Solid Edge part; units mm, degrees
sketch "Sketch1" plane through (0, 0, 0) normal (0, 0, 1) x (1, 0, 0)
  circle A0 centre (0, 0) radius 4.25
extrude "Protrusion1" add sketch "Sketch1" along normal blind 5
sketch "Sketch2" plane through (0, 0, 0) normal (0, 0, -1) x (1, 0, 0)
  circle A0 centre (0, 0) radius 2.5
extrude "Protrusion2" add sketch "Sketch2" along normal blind 20
sketch "Sketch3" plane through (0, 0, -20) normal (0, 0, -1) x (1, 0, 0)
  circle A0 centre (0, 0) radius 2.4997
extrude "Cutout1" cut sketch "Sketch3" against normal blind 19.98 flip side to cut
chamfer "Chamfer_1" distance 0.375 angle 45 1 edges at (-2.4997, 0, -20)
sketch "Sketch4" plane through (0, 0, 5) normal (0, 0, 1) x (1, 0, 0)
  line L0 (-1.1547, 2) -> (1.1547, 2)
  line L1 (2.3094, 0) -> (1.1547, 2)
  line L2 (1.1547, -2) -> (2.3094, 0)
  line L3 (-1.1547, -2) -> (1.1547, -2)
  line L4 (-2.3094, 0) -> (-1.1547, -2)
  line L5 (-1.1547, 2) -> (-2.3094, 0)
extrude "Cutout2" cut sketch "Sketch4" against normal blind 2.5
properties part number "24104804"
Can you work these out from the model? Positions are in its coordinate system, mm. A direction names the side the tool comes from. Give positions to 0.01 mm unless a question says otherwise; leave off trailing zeros. Order: outer loops, then holes, each group sorted by start corner. A loop starts at its lowest first (then second) coordinate and runs counter-clockwise, first axis right, second up. Notation, with made-up numbers: M 88.5,-31 L 122.5,-31 A36 cw 122.5,3 Z; hole C 4.5,33.25 d10. An arc over 180 degrees is marked long. Write item = value, one per line. Start each with the question number.
Q1. Will these pins go through, and if not, where does the flat tip stop? pin 1 Ø1.5 at (y, z) = (1.5, -11.5) entering from +X; pin 2 Ø4 at (x, z) = (3, -5) entering from +Y; pin 3 Ø4 at (x, z) = (1, -16) entering from +Y.
Q2. For faces 5 (the flat face through (0, 2, 4)), 6 (the cylindrical face through (-2, 1.5, -10)), 7 (the flat face through (0, 0, -20)), which set-ups out of +Z, -Z, +X, -X, +Y, -Y let a thin tool reach every point of the face, with its end or its side?
Q3. Suppose I cut it at C-C (y = 3). Write out the boundary of the cut face in (x, z), plus the area to 3 significant figures.
Q4. Suppose I cut it at D-D (x = 3.25). Write out the boundary of the cut face in (y, z).
Q5. I need wall thicknesses on probe 1 along Z at (x, y) = (-1.5, 3); probe 2 along Z at (x, y) = (0.5, 1.25); probe 3 along Y at (x, z) = (3.75, 1.5). Which ranges of each line are inside material? Lowest first, please. Write a range as [from, to].
Q6. We'd pull the mould along X, two halves only. Please class faces 1 (the flat face through (0, 0, 2.5)), 2 (the flat face through (2, -1, 5)), 3 (the cylindrical face through (2.285, -3.584, 2.465)), 4 (the flat face through (1.724, -1.014, 3.768)): pulls with the +X half, pulls with the -X half, needs draft (parallel to the pull), parting line crosses it, or undercut.
Q7. Suppose I cut it at B-B (z = 0.5). Write out the boundary of the cut face in (x, y), plus the area to 3 significant figures.
Check result:
q1.pin_1 = 2.38
q1.pin_2 = 2.29
q1.pin_3 = 2.5
q2.face_5 = +Z
q2.face_6 = -Z
q2.face_7 = -Z, +X, -X, +Y, -Y
q3.outline = M -3.01,0 L 3.01,0 L 3.01,5 L -3.01,5 Z
q3.area = 30.1 mm2
q4.outline = M -2.74,0 L 2.74,0 L 2.74,5 L -2.74,5 Z
q5.probe_1 = [0, 5]
q5.probe_2 = [-20, 2.5]
q5.probe_3 = [-2, 2]
q6.face_1 = undercut
q6.face_2 = needs draft
q6.face_3 = parting line crosses it
q6.face_4 = undercut
q7.outline = C 0,0 d8.5
q7.area = 56.7 mm2
